Verification items for the finished model (mm, model axes). Face numbers are marked on the shaded views. A direction names the side the tool comes from. Round coordinates to 2 decimals unless told otherwise and drop trailing zeros. Write each loop counter-clockwise with the first axis right and the second up, starting at its lowest first coordinate (ties: lowest second). Pieces come first, ordered by that corner, then holes. Notation, with made-up numbers: (-8.75, 36) -> (16.25, 36) arc R27 ccw to (16.25, 53) -> close; hole circle Ø5 at (81.25, 59). An arc over 180 degrees is marked (long way). Answer as a JSON object with one key per item and string values. Group by question number.
(1) Draft check along X on the marked faces 1, 2, 3 and 4. Enter one of: released by +X, released by -X, zero draft, split by the parting line, or undercut.
(2) Sectioned sample at C-C on x = 38. Record the cut outline in (y, z), and give its area (3 significant figures).
(3) Gauge pin test, flat ends, axial feed: pin 1 Ø6 at (x, y) = (23, 2.5) entering from -Z; pin 2 Ø1.9 at (y, z) = (6.5, 22) entering from +X (3 decimals); pin 3 Ø1 at (x, y) = (150, 3.5) entering from +Z; pin 4 Ø4 at (y, z) = (4, 21) entering from -X. Record the tip position at first contact, or that the pin passes through.
(4) Scan lines: L1, parallel to X at y = 1.25, z = 11 (3 decimals); L2, parallel to Z at x = 17, y = 3.25; L3, parallel to X at y = 5, z = 6.5 (3 decimals). Record each from-to range of solid material in increasing order. Write a range as from..to.
(5) Sectioned sample at B-B on z = 9.5. Record the cut outline in (x, y) (3 decimals), and give its area (3 significant figures).
(6) Set-up check for the marked faces 5, 6, 7, 8 and 9: record each of +Z, -Z, +X, -X, +Y, -Y from which the full face is reachable in a straight line by a thin tool's end or side.
(7) Sectioned sample at A-A on x = 122. Record the cut outline in (y, z).
(8) Sectioned sample at D-D on z = 21.75. Record the cut outline in (x, y) (3 decimals).
Autodesk Inventor part; units mm, degrees
ref_plane "YZ Plane" through (0, 0, 0) normal (1, 0, 0) x (0, 1, 0)
ref_plane "XZ Plane" through (0, 0, 0) normal (0, 1, 0) x (-1, 0, 0)
ref_plane "XY Plane" through (0, 0, 0) normal (0, 0, 1) x (1, 0, 0)
sketch "Sketch1" plane through (0, 0, 0) normal (0, 0, 1) x (1, 0, 0)
  line L0 (0, 0) -> (152.4, 0)
  line L1 (152.4, 0) -> (152.4, 12.7)
  line L2 (152.4, 12.7) -> (0, 12.7)
  line L3 (0, 12.7) -> (0, 0)
  dimension "d0" = 152.4
  dimension "d1" = 12.7
sketch "Sketch1 outline for Extrusion1" plane through (0, 0, 0) normal (0, 0, 1) x (1, 0, 0)
  line L0 (0, 12.7) -> (0, 0)
  line L1 (152.4, 12.7) -> (0, 12.7)
  line L2 (152.4, 0) -> (152.4, 12.7)
  line L3 (0, 0) -> (152.4, 0)
extrude "Extrusion1" add sketch "Sketch1 outline for Extrusion1" along normal blind 6.35
chamfer "Chamfer1" distance 3.175 angle 45 2 edges at (152.4, 12.7, 3.175) (152.4, 0, 3.175)
sketch "Sketch2" plane through (0, 0, 6.35) normal (0, 0, 1) x (1, 0, 0)
  line L0 (0, 0) -> (149.225, 0)
  line L1 (149.225, 12.7) -> (0, 12.7)
  line L2 (15.570231, 0) -> (3.175, 0)
  line L3 (3.175, 0) -> (3.175, 12.7)
  line L4 (3.175, 12.7) -> (15.570231, 12.7)
  line L5 (15.570231, 12.7) -> (15.570231, 0)
  point P0 (3.175, 0)
sketch "Sketch2 outline for Extrusion2" plane through (0, 0, 6.35) normal (0, 0, 1) x (1, 0, 0)
  line L0 (15.570231, 0) -> (3.175, 0)
  line L1 (3.175, 0) -> (3.175, 12.7)
  line L2 (3.175, 12.7) -> (15.570231, 12.7)
  line L3 (15.570231, 12.7) -> (15.570231, 0)
extrude "Extrusion2" add sketch "Sketch2 outline for Extrusion2" along normal blind 12.7
fillet "Fillet1" radius 6.35 2 edges at (9.3726, 12.7, 19.05) (9.3726, 0, 19.05)
shell "Shell1" thickness 2.54 removed faces 1 at (15.570231, 8.466667, 10.5834)
sketch "Sketch3" plane through (0, 0, 6.35) normal (0, 0, 1) x (1, 0, 0)
  line L0 (0, 0) -> (149.225, 0)
  line L1 (149.225, 12.7) -> (0, 12.7)
  line L2 (149.225, 0) -> (73.440725, 0)
  line L3 (73.440725, 0) -> (73.440725, 12.7)
  line L4 (73.440725, 12.7) -> (149.225, 12.7)
  line L5 (149.225, 12.7) -> (149.225, 0)
sketch "Sketch3 outline for Extrusion3" plane through (0, 0, 6.35) normal (0, 0, 1) x (1, 0, 0)
  line L0 (149.225, 0) -> (73.440725, 0)
  line L1 (73.440725, 0) -> (73.440725, 12.7)
  line L2 (73.440725, 12.7) -> (149.225, 12.7)
  line L3 (149.225, 12.7) -> (149.225, 0)
extrude "Extrusion3" add sketch "Sketch3 outline for Extrusion3" along normal blind 19.05
sketch "Sketch4" plane through (149.225, 0, 6.35) normal (1, 0, 0) x (0, 0, -1)
  line L0 (-19.05, 12.7) -> (-19.05, 0)
  circle A0 centre (-19.05, 6.35) radius 6.35
  point P0 (6.35, 0)
sketch "Sketch4 outline for Extrusion4" plane through (149.225, 0, 6.35) normal (1, 0, 0) x (0, 0, -1)
  circle A0 centre (-19.05, 6.35) radius 6.35
extrude "Extrusion4" cut sketch "Sketch4 outline for Extrusion4" against normal blind 19.05
properties part number "Lolipop"
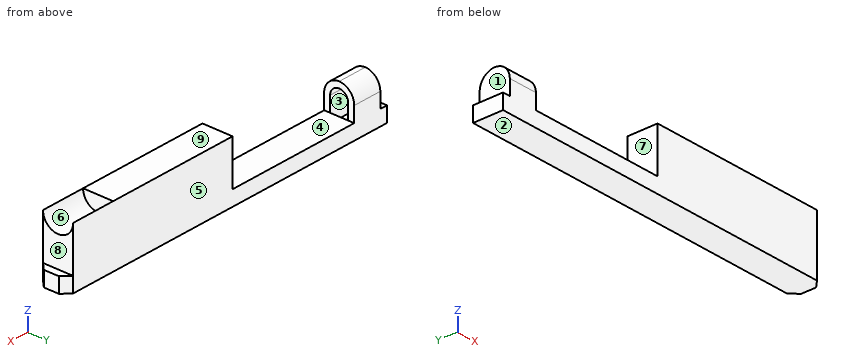
Computed values:
{
 "1": {"face 1": "released by -X", "face 2": "zero draft", "face 3": "undercut", "face 4": "undercut"},
 "2": {"outline": "(0, 0) -> (12.7, 0) -> (12.7, 6.35) -> (0, 6.35) -> close; hole (2.54, 2.54) -> (10.16, 2.54) -> (10.16, 3.81) -> (2.54, 3.81) -> close", "area": "71.0 mm2"},
 "3": {"pin 1": "z = 0", "pin 2": "x = 130.175", "pin 3": "z = 6.35", "pin 4": "x = 73.44"},
 "4": {"L1": "3.175..15.57, 73.441..149.225", "L2": "0..2.54, 3.81..6.35", "L3": "3.175..5.715, 73.441..149.225"},
 "5": {"outline": "(3.175, 0) -> (15.57, 0) -> (15.57, 2.54) -> (5.715, 2.54) -> (5.715, 10.16) -> (15.57, 10.16) -> (15.57, 12.7) -> (3.175, 12.7) -> close; (73.441, 0) -> (149.225, 0) -> (149.225, 12.7) -> (73.441, 12.7) -> close", "area": "1,040 mm2"},
 "6": {"face 5": "+Z, -Z, +X, -X, +Y", "face 6": "+Z, +X", "face 7": "+Z, +Y, -Y", "face 8": "+Z, +X, +Y, -Y", "face 9": "+Z, +X, -X, +Y, -Y"},
 "7": {"outline": "(0, 0) -> (12.7, 0) -> (12.7, 25.4) -> (0, 25.4) -> close; hole (2.54, 2.54) -> (10.16, 2.54) -> (10.16, 3.81) -> (2.54, 3.81) -> close"},
 "8": {"outline": "(73.441, 0) -> (149.225, 0) -> (149.225, 1.154) -> (130.175, 1.154) -> (130.175, 11.546) -> (149.225, 11.546) -> (149.225, 12.7) -> (73.441, 12.7) -> close"}
}
